from build123d import *

# Parameters (mm, degrees)
BOSS_EXTRUDE1_DEPTH = 5
SKETCH8_W           = 50
SKETCH8_H           = 70
CUT_EXTRUDE2_DEPTH  = 50
BOSS_EXTRUDE2_START = -30
SKETCH6_W           = 3
SKETCH6_H           = 2
SKETCH6_H_2         = 3
SKETCH6_W_2         = 10
BOSS_EXTRUDE2_DEPTH = 60
BOSS_EXTRUDE3_START = -30
SKETCH7_W           = 46
SKETCH7_H           = 5
BOSS_EXTRUDE3_DEPTH = 3
SKETCH11_W          = 46
SKETCH11_H          = 63
BOSS_EXTRUDE4_DEPTH = 5
BOSS_EXTRUDE6_REACH = 56.109
SKETCH13_W          = 51.830863245
SKETCH13_H          = 5.290230228
BOSS_EXTRUDE7_DEPTH = 5
BOSS_EXTRUDE8_START = 5.021523682
BOSS_EXTRUDE8_DEPTH = 1.000000021


# Read off the part's stored shape, not the designer's step: Boss-Extrude8
with BuildPart() as part:
    # Sketch4 → Boss-Extrude1 (new body)
    with BuildSketch(Plane(origin=(0, 0, 0), x_dir=(0, 1, 0), z_dir=(0, 0, 1))):
        Polygon((-39.75, -29.75), (-14.905444566, -29.75), (-16.637495374, -26.75), (0.24999995, -26.75), (17.137495374, -26.75), (15.405444566, -29.75), (39.75, -29.75), (39.75, -10), (36.75, -10), (36.75, 10), (39.75, 10), (39.75, 29.75), (15.405444566, 29.75), (17.137495374, 26.75), (0.250000065, 26.75), (-16.637495374, 26.75), (-14.905444566, 29.75), (-39.75, 29.75), (-39.75, 10), (-36.75, 10), (-36.75, -10), (-39.75, -10), align=None)
    extrude(amount=BOSS_EXTRUDE1_DEPTH)

    # Sketch8 → Cut-Extrude2 (cut)
    with BuildSketch(Plane(origin=(0, 0, 0), x_dir=(1, 0, 0), z_dir=(0, 0, -1))):
        Rectangle(SKETCH8_W, SKETCH8_H)
    extrude(amount=-CUT_EXTRUDE2_DEPTH, mode=Mode.SUBTRACT)



with BuildPart() as body_2:
    # Sketch6 → Boss-Extrude2 (new body)
    with BuildSketch(Plane(origin=(0, -0.558315077, -3.166362145), x_dir=(1, 0, 0), z_dir=(0, -0.9848077530122069, 0.1736481776669375)).offset(BOSS_EXTRUDE2_START)):
        with Locations((-21.528635138, 15.236732087)):
            Rectangle(SKETCH6_W, SKETCH6_H)
        with Locations((-21.528635138, 17.736732087)):
            Rectangle(SKETCH6_W, SKETCH6_H_2)
        with Locations((-15.028635138, 17.736732087)):
            Rectangle(SKETCH6_W_2, SKETCH6_H_2)
        with Locations((21.471364862, 15.236732087)):
            Rectangle(SKETCH6_W, SKETCH6_H)
        with Locations((21.471364862, 17.736732087)):
            Rectangle(SKETCH6_W, SKETCH6_H_2)
        with Locations((14.971364862, 17.736732087)):
            Rectangle(SKETCH6_W_2, SKETCH6_H_2)
    extrude(amount=BOSS_EXTRUDE2_DEPTH)



with BuildPart() as body_3:
    # Sketch7 → Boss-Extrude3 (new body)
    with BuildSketch(Plane(origin=(0, 0, 0), x_dir=(-1, 0, 0), z_dir=(0, 0.9848077530122069, -0.1736481776669375)).offset(BOSS_EXTRUDE3_START)):
        with Locations((0.028635138, 13.521523703)):
            Rectangle(SKETCH7_W, SKETCH7_H)
    extrude(amount=-BOSS_EXTRUDE3_DEPTH)


with BuildPart() as body_2_1:
    add(body_2.part)

    add(body_3.part)  # Boss-Extrude4 merges body 3
    # Sketch11 → Boss-Extrude4 (add)
    with BuildSketch(Plane(origin=(0, 1.913867506, 10.854081993), x_dir=(1, 0, 0), z_dir=(0, -0.17364817766693746, -0.9848077530122068))):
        with Locations((-0.028635138, 1.5)):
            Rectangle(SKETCH11_W, SKETCH11_H)
    extrude(amount=BOSS_EXTRUDE4_DEPTH)


with BuildPart() as part_1:
    add(part.part)

    add(body_2_1.part)  # Boss-Extrude6 merges body 2
    # Boss-Extrude6: up to this plane
    boss_extrude6_end = Plane(origin=(22.971364862, 32.326340985, 10.568675428), z_dir=(0, 0.17364817766693744, 0.9848077530122069))
    # Sketch12 → Boss-Extrude6 (add, up to the surface)
    with BuildSketch(Plane(origin=(0, 0, 0), x_dir=(1, 0, 0), z_dir=(0, 0, -1)), mode=Mode.PRIVATE) as boss_extrude6_sk1:
        Polygon((-25, -32.326340985), (-22.25188492, -32.326340985), (-22.25188492, 27.03466657), (22.017654552, 27.03466657), (22.017654552, -32.326340985), (25, -32.326340985), (25, 35), (-25, 35), align=None)
    boss_extrude6_tool1 = split(extrude(boss_extrude6_sk1.sketch, amount=-BOSS_EXTRUDE6_REACH, mode=Mode.PRIVATE), bisect_by=boss_extrude6_end, keep=Keep.BOTH, mode=Mode.PRIVATE)
    add(boss_extrude6_tool1.solids().sort_by_distance((-23.625942, 31.487721, 0))[0])

    # Sketch13 → Boss-Extrude7 (add)
    with BuildSketch(Plane(origin=(0, 0, 0), x_dir=(1, 0, 0), z_dir=(0, 0, -1))):
        with Locations((-0.078348401, -32.848959795)):
            Rectangle(SKETCH13_W, SKETCH13_H)
    extrude(amount=-BOSS_EXTRUDE7_DEPTH)

    # Boss-Extrude8 outline → Boss-Extrude8 (add)
    # profile 1 of 3: a face of its own
    with BuildSketch(Plane(origin=(0, 0, 0), x_dir=(1, 0, 0), z_dir=(0, 0.1736481776669375, 0.9848077530122069)).offset(BOSS_EXTRUDE8_START)):
        with BuildLine():
            add(Edge.make_bspline(
                [(-10.467851841, 5.945152171), (-10.986974105, 5.93651447), (-11.500854153, 5.896229421), (-12.498790484, 5.635612757), (-12.985546819, 5.414483257), (-13.797961559, 4.74423563), (-14.118849525, 4.313672985), (-14.500878838, 3.342927953), (-14.563491586, 2.813042118), (-14.576316895, 2.28783257)],
                knots=[0, 0, 0, 0, 0.25, 0.25, 0.5, 0.5, 0.75, 0.75, 1, 1, 1, 1], degree=3))
            add(Edge.make_bspline(
                [(-14.576316895, 2.28783257), (-14.564248114, 1.730329849), (-14.485127057, 1.171617147), (-14.041607684, 0.154100247), (-13.697450783, -0.299455445), (-12.861318405, -1.029274155), (-12.357191638, -1.292181087), (-11.287857522, -1.614507239), (-10.731412411, -1.666616468), (-10.173846939, -1.678699083)],
                knots=[0, 0, 0, 0, 0.25, 0.25, 0.5, 0.5, 0.75, 0.75, 1, 1, 1, 1], degree=3))
            Line((-10.173846939, -1.678699083), (-8.574561652, -1.678699083))
            Line((-8.574561652, -1.678699083), (-8.574561652, -6.382777516))
            Line((-8.574561652, -6.382777516), (-7.114675242, -6.382777516))
            Line((-7.114675242, -6.382777516), (-7.114675242, 5.945152171))
            Line((-7.114675242, 5.945152171), (-10.467851841, 5.945152171))
        make_face()
        with BuildLine():
            Line((-8.574561652, -0.381022274), (-10.075000463, -0.381022274))
            add(Edge.make_bspline(
                [(-10.075000463, -0.381022274), (-10.454019642, -0.376067015), (-10.82957333, -0.347620207), (-11.563501324, -0.174272567), (-11.922431464, -0.026106182), (-12.530252018, 0.44277106), (-12.769732325, 0.751236277), (-13.058396455, 1.452245522), (-13.106849265, 1.837560064), (-13.116430485, 2.219400395)],
                knots=[0, 0, 0, 0, 0.25, 0.25, 0.5, 0.5, 0.75, 0.75, 1, 1, 1, 1], degree=3))
            add(Edge.make_bspline(
                [(-13.116430485, 2.219400395), (-13.111547413, 2.5782319), (-13.069607652, 2.936381873), (-12.8109443, 3.606784644), (-12.593110897, 3.90761083), (-11.721692221, 4.542687822), (-10.970699083, 4.634581597), (-10.252417214, 4.647475362)],
                knots=[0, 0, 0, 0, 0.25, 0.25, 0.5, 0.5, 1, 1, 1, 1], degree=3))
            Line((-10.252417214, 4.647475362), (-8.574561652, 4.647475362))
            Line((-8.574561652, 4.647475362), (-8.574561652, -0.381022274))
        make_face(mode=Mode.SUBTRACT)
    # profile 2 of 3: a face of its own
    with BuildSketch(Plane(origin=(0, 0, 0), x_dir=(1, 0, 0), z_dir=(0, 0.1736481776669375, 0.9848077530122069)).offset(BOSS_EXTRUDE8_START)):
        Polygon((14.783620913, 4.647475362), (14.783620913, 5.945152171), (6.186512052, 5.945152171), (6.186512052, 4.647475362), (9.755123278, 4.647475362), (9.755123278, -6.382777516), (11.215009688, -6.382777516), (11.215009688, 4.647475362), align=None)
    # profile 3 of 3: a face of its own
    with BuildSketch(Plane(origin=(0, 0, 0), x_dir=(1, 0, 0), z_dir=(0, 0.1736481776669375, 0.9848077530122069)).offset(BOSS_EXTRUDE8_START)):
        Polygon((5.699883249, -6.382777516), (0.945114315, 5.945152171), (-0.55785902, 5.945152171), (-5.330369629, -6.382777516), (-3.723480768, -6.382777516), (-2.423269434, -2.976375892), (2.868818804, -2.976375892), (4.082856287, -6.382777516), align=None)
        with BuildLine():
            Line((0.202498485, 4.485265761), (0.23544731, 4.485265761))
            add(Edge.make_bspline(
                [(0.23544731, 4.485265761), (0.247945589, 4.41509498), (0.260444435, 4.344921063), (0.273754544, 4.274899734), (0.287066266, 4.20486992), (0.301165705, 4.134968363), (0.317053985, 4.065477793), (0.34874631, 3.92686507), (0.391135692, 3.790647481), (0.438209312, 3.65647608)],
                knots=[0, 0, 0, 0, 0.250067921, 0.250067921, 0.250067921, 0.500190861, 0.500190861, 0.500190861, 1, 1, 1, 1], degree=3))
            Line((0.438209312, 3.65647608), (2.389793575, -1.678699083))
            Line((2.389793575, -1.678699083), (-1.94677873, -1.678699083))
            Line((-1.94677873, -1.678699083), (0.014943634, 3.65647608))
            add(Edge.make_bspline(
                [(0.014943634, 3.65647608), (0.036185093, 3.724160229), (0.057270848, 3.791932402), (0.075717575, 3.860431029), (0.094170953, 3.928954356), (0.110345138, 3.998113348), (0.124780214, 4.067594296), (0.153586161, 4.206247155), (0.177650794, 4.345849154), (0.202498485, 4.485265761)],
                knots=[0, 0, 0, 0, 0.250210129, 0.250210129, 0.250210129, 0.500538862, 0.500538862, 0.500538862, 1, 1, 1, 1], degree=3))
        make_face(mode=Mode.SUBTRACT)
    extrude(amount=BOSS_EXTRUDE8_DEPTH)


solid = part_1.part
Here's how the part is built. I have some questions about the finished solid (model axes, mm). A direction names the side the tool comes from. Give positions to 0.01 mm unless a question says otherwise; leave off trailing zeros. Order: outer loops, then holes, each group sorted by start corner. A loop starts at its lowest first (then second) coordinate and runs counter-clockwise, first axis right, second up. Notation, with made-up numbers: (80.5, -11.75) -> (90.5, -11.75) arc R11 ccw to (90.5, -2.75) -> close; hole circle Ø11 at (79.25, -15.5). An arc over 180 degrees is marked (long way). One line per item, written item: value. Start each with the question number.
1. Imagine slicing it at A-A, the plane x = -16. List the corners of the cut face in (y, z) for me.
2. Imagine slicing it at D-D, the plane z = 17. List the corners of the cut face in (x, y) for me.
3. Imagine slicing it at B-B, the plane y = -32.5. List the corners of the cut face in (x, z) for me.
4. I need wall thicknesses on probe 1 along X at (y, z) = (12, 10); probe 2 along X at (y, z) = (-19, 17); probe 3 along X at (y, z) = (-21.5, 14.5). Which ranges of each line are inside material? Lowest first, please. Write a range as from..to.
5. We'd pull the mould along X, two halves only. Please class faces 4 (the face through (-2.91, 0.83, 5.45)), 5 (the face through (25, -8, 12)), 6 (the face through (23, 32.326, 8)), 7 (the face through (9.971, 3, 14)): released by +X, released by -X, zero draft, split by the parting line, or undercut.
6. Imagine slicing it at C-C, the plane z = 9.75. List the corners of the cut face in (x, y) for me, plus the area to 3 significant figures.
7. Will these pins go through, and if not, where does the flat tip stop? pin 1 Ø1.5 at (x, z) = (23, 8) entering from +Y; pin 2 Ø12 at (x, y) = (15.5, 20.5) entering from +Z; pin 3 Ø10 at (y, z) = (-7, 18.5) entering from -X.
8. For faces 1 (the face through (-24, 32.326, 8)), 2 (the face through (0, -27.035, 5)), 3 (the face through (19.971, 3, 12)), which set-ups out of +Z, -Z, +X, -X, +Y, -Y let a thin tool reach every point of the face, with its end or its side?
Values follow:
1. outline: (-39.75, 0) -> (-27.03, 0) -> (-27.03, 10.88) -> (30.2, 0.79) -> (30.2, 0) -> (39.75, 0) -> (39.75, 5) -> (31.34, 5) -> (31.46, 5.64) -> (-27.03, 15.96) -> (-27.03, 17.99) -> (31.81, 7.61) -> (32.33, 10.57) -> (-35, 22.44) -> (-35, 5) -> (-39.75, 5) -> close
2. outline: (-25, -35) -> (25, -35) -> (25, -4.15) -> (9.97, -4.15) -> (9.97, -21.42) -> (19.97, -21.42) -> (19.97, -27.03) -> (-20.03, -27.03) -> (-20.03, -21.42) -> (-10.03, -21.42) -> (-10.03, -4.15) -> (-25, -4.15) -> close
3. outline: (-29.75, 0) -> (29.75, 0) -> (29.75, 5) -> (25, 5) -> (25, 22) -> (-25, 22) -> (-25, 5) -> (-29.75, 5) -> close
4. probe 1: x = -25..-20.03, 19.97..25
4. probe 2: x = -25..-10.03, 9.97..25
4. probe 3: x = -25..25
5. face 4: undercut
5. face 5: released by +X
5. face 6: zero draft
5. face 7: undercut
6. outline: (-25, -35) -> (25, -35) -> (25, 32.33) -> (22.02, 32.33) -> (22.02, 32.18) -> (9.97, 32.18) -> (9.97, 19.69) -> (19.97, 19.69) -> (19.97, 8.18) -> (-20.03, 8.18) -> (-20.03, 19.69) -> (-10.03, 19.69) -> (-10.03, 32.18) -> (-22.25, 32.18) -> (-22.25, 32.33) -> (-25, 32.33) -> close; hole (-22.25, -27.03) -> (22.02, -27.03) -> (22.02, -20.62) -> (-22.25, -20.62) -> close
6. area: 2,370 mm2
7. pin 1: stops at y = 32.33
7. pin 2: stops at z = 13.71
7. pin 3: stops at x = -25
8. face 1: +Z, +X, -X, +Y
8. face 2: -Z
8. face 3: none
